```python
from build123d import *

# Parameters (mm, degrees)
SKETCH1_R           = 6
BOSS_EXTRUDE1_DEPTH = 3.45
SKETCH2_W           = 3.175
SKETCH2_H           = 20
BOSS_EXTRUDE2_DEPTH = 21.55
SKETCH3_W           = 25
SKETCH3_H           = 3.675
BOSS_EXTRUDE3_DEPTH = 12.65
FILLET1_R           = 5
SKETCH5_R           = 1.5
CUT_EXTRUDE1_DEPTH  = 12.65
SKETCH6_R           = 3
CUT_EXTRUDE2_DEPTH  = 2.5
FILLET2_R           = 5


with BuildPart() as part:
    # Sketch1 → Boss-Extrude1 (new body)
    with BuildSketch(Plane.XY):
        with BuildLine():
            Line((0, 10), (-12.5, 10))
            Line((-12.5, 10), (-12.5, -10))
            Line((-12.5, -10), (0, -10))
            ThreePointArc((0, -10), (10, 0), (0, 10))
        make_face()
        with Locations(Location((0, 0, 0), (0, 0, 180))):
            Circle(SKETCH1_R, mode=Mode.SUBTRACT)
    extrude(amount=BOSS_EXTRUDE1_DEPTH)

    # Sketch2 → Boss-Extrude2 (add)
    with BuildSketch(Plane.XY.offset(3.45)):
        with Locations((-10.9125, 0)):
            Rectangle(SKETCH2_W, SKETCH2_H)
    extrude(amount=BOSS_EXTRUDE2_DEPTH)

    # Sketch3 → Boss-Extrude3 (add)
    with BuildSketch(Plane.ZY.offset(12.5)):
        with Locations((12.5, 8.1625)):
            Rectangle(SKETCH3_W, SKETCH3_H)
        with Locations((12.5, -8.1625)):
            Rectangle(SKETCH3_W, SKETCH3_H)
    extrude(amount=BOSS_EXTRUDE3_DEPTH)

    # Fillet1
    fillet1_edges = [part.edges().sort_by_distance(p)[0] for p in [
        (-9.325, 10, 14.225),
        (-9.325, -10, 14.225),
    ]]
    fillet(fillet1_edges, radius=FILLET1_R)

    # Sketch5 → Cut-Extrude1 (cut)
    with BuildSketch(Plane(origin=(-9.325, 0, 0), x_dir=(0, 0, -1), z_dir=(1, 0, 0))):
        with Locations(Location((-19, 0, 0), (0, 0, 90))):
            Circle(SKETCH5_R)
        with Locations(Location((-9, 0, 0), (0, 0, 90))):
            Circle(SKETCH5_R)
    extrude(amount=-CUT_EXTRUDE1_DEPTH, mode=Mode.SUBTRACT)

    # Sketch6 → Cut-Extrude2 (cut)
    with BuildSketch(Plane(origin=(-9.325, 0, 0), x_dir=(0, 0, -1), z_dir=(1, 0, 0))):
        with Locations(Location((-19, 0, 0), (0, 0, 90))):
            Circle(SKETCH6_R)
        with Locations(Location((-9, 0, 0), (0, 0, 90))):
            Circle(SKETCH6_R)
    extrude(amount=-CUT_EXTRUDE2_DEPTH, mode=Mode.SUBTRACT)

    # Fillet2
    # the kernel refuses this fillet: 5 mm, written as the material it takes off along each edge
    with BuildSketch(Plane(origin=(-25.15, 10, 37.05310515), x_dir=(1, 0, 0), z_dir=(0, 0, -1))) as fillet2_piece_1:
        with BuildLine():
            CenterArc((4.82124206, 5), FILLET2_R, 195.366952798, 74.633047202)
            Line((0, 3.675), (-0.096424841, 3.6485))
            ThreePointArc((-0.096424841, 3.6485), (-0.1, 1.8375), (-0.1, 0))
            Line((-0.1, 0), (0, -0.1))
            Line((0, -0.1), (4.82124206, -0.1))
            Line((4.82124206, -0.1), (4.82124206, 0))
        make_face()
    extrude(amount=49.106210299, mode=Mode.SUBTRACT)
    with BuildSketch(Plane(origin=(-25.15, -10, 37.05310515), x_dir=(1, 0, 0), z_dir=(0, 0, -1))) as fillet2_piece_2:
        with BuildLine():
            CenterArc((4.82124206, -5), FILLET2_R, 90, 74.633047202)
            Line((0, -3.675), (-0.096424841, -3.6485))
            ThreePointArc((-0.096424841, -3.6485), (-0.1, -1.8375), (-0.1, 0))
            Line((-0.1, 0), (0, 0.1))
            Line((0, 0.1), (4.82124206, 0.1))
            Line((4.82124206, 0.1), (4.82124206, 0))
        make_face()
    extrude(amount=49.106210299, mode=Mode.SUBTRACT)


solid = part.part
```
Design review of the part built by this model. Coordinates are the model's own, in mm. A direction names the side the tool comes from. Round coordinates to 2 decimals unless told otherwise and drop trailing zeros. Write each loop counter-clockwise with the first axis right and the second up, starting at its lowest first coordinate (ties: lowest second). Pieces come first, ordered by that corner, then holes.
Item 1: We need section C-C on x = 2. Write out the cut boundary in (y, z), and give its area (3 significant figures).
Item 2: We need section A-A on z = 19. Write out the cut boundary in (x, y) (3 decimals).
Item 3: We need section D-D on z = 4. Write out the cut boundary in (x, y) (3 decimals), and give its area (3 significant figures).
Item 4: For probe 1 along Z at (x, y) = (-12.3, 0); probe 2 along Z at (x, y) = (-10.5, 0); probe 3 along X at (y, z) = (-1.5, 20) (3 decimals), list the stretches that pass through material, from the lowest coordinate up.
Item 5: Clearance check with flat-ended pins moving along their axes: pin 1 Ø5 at (y, z) = (0, 19) entering from -X; pin 2 Ø4 at (y, z) = (-5, 21.5) entering from +X (3 decimals); pin 3 Ø5 at (y, z) = (0, 19) entering from +X (3 decimals). State where each tip first meets the part, or that it passes through.
Item 6: We need section B-B on y = 0. Write out the cut boundary in (x, z) (3 decimals).
Item 7: The part is to be moulded in two halves that separate along Z. For faces 1 (the cylindrical face through (-12.158, 0.806, 20.265)), 2 (the flat face through (-7, 0, 0)), 3 (the flat face through (-12, 0, 25)), 4 (the cylindrical face through (-10.751, -8.496, 14.376)), say which applies: +Z half, -Z half, draft (parallel to the pull), parting line (faces both ways), or undercut.
Item 8: For faces 5 (the flat face through (-12.5, 0, 12)), 6 (the flat face through (-9.325, 0, 14)), 7 (the cylindrical face through (-10.56, -0.65, 16.07)), 8 (the cylindrical face through (-5.723, -1.802, 1.701)), 9 (the cylindrical face through (-10.751, 8.496, 14.376)), list the 3-axis set-ups (+Z, -Z, +X, -X, +Y, -Y) from which the entire face can be reached by the end or side of a thin tool; tool diameter is ignored.
Returned:
1. outline: (-9.8, 0) - (-5.66, 0) - (-5.66, 3.45) - (-9.8, 3.45) - close; (5.66, 0) - (9.8, 0) - (9.8, 3.45) - (5.66, 3.45) - close
1. area: 28.6 mm2
2. outline: (-25.15, -6.325) arc R5 ccw to (-20.329, -10) - (-14.325, -10) arc R5 ccw to (-9.325, -5) - (-9.325, -3) - (-11.825, -3) - (-11.825, -1.5) - (-12.5, -1.5) - (-12.5, -6.325) - close; (-25.15, 6.325) - (-12.5, 6.325) - (-12.5, 1.5) - (-11.825, 1.5) - (-11.825, 3) - (-9.325, 3) - (-9.325, 5) arc R5 ccw to (-14.325, 10) - (-20.329, 10) arc R5 ccw to start
3. outline: (-25.15, -6.325) arc R5 ccw to (-20.329, -10) - (-14.325, -10) arc R5 ccw to (-9.325, -5) - (-9.325, 5) arc R5 ccw to (-14.325, 10) - (-20.329, 10) arc R5 ccw to (-25.15, 6.325) - (-12.5, 6.325) - (-12.5, -6.325) - close
3. area: 136 mm2
4. probe 1: z = 0 to 7.5, 10.5 to 17.5, 20.5 to 25
4. probe 2: z = 0 to 6, 12 to 16, 22 to 25
4. probe 3: x = -12.5 to -11.825
5. pin 1: stops at x = -12.5
5. pin 2: stops at x = -9.325
5. pin 3: stops at x = -11.825
6. outline: (-12.5, 0) - (-6, 0) - (-6, 3.45) - (-9.325, 3.45) - (-9.325, 6) - (-11.825, 6) - (-11.825, 7.5) - (-12.5, 7.5) - close; (-12.5, 10.5) - (-11.825, 10.5) - (-11.825, 12) - (-9.325, 12) - (-9.325, 16) - (-11.825, 16) - (-11.825, 17.5) - (-12.5, 17.5) - close; (-12.5, 20.5) - (-11.825, 20.5) - (-11.825, 22) - (-9.325, 22) - (-9.325, 25) - (-12.5, 25) - close; (6, 0) - (10, 0) - (10, 3.45) - (6, 3.45) - close
7. face 1: undercut
7. face 2: -Z half
7. face 3: +Z half
7. face 4: draft
8. face 5: +Z, -Z, -X
8. face 6: +Z, +X, +Y, -Y
8. face 7: +X
8. face 8: +Z, -Z
8. face 9: +Z, +X, +Y
